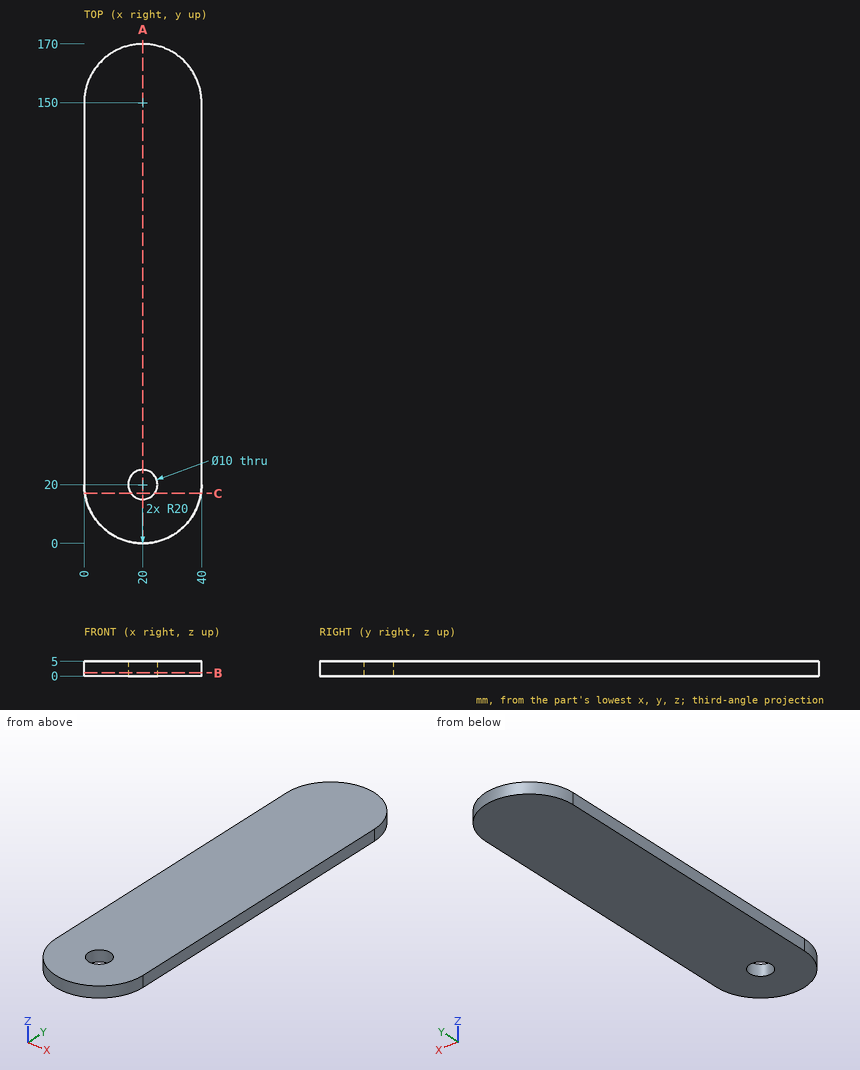
Print and shaded views of the part. All mm, measured from the part's lowest x, y and z. Coordinates: 2 decimals unless noted, no trailing zeros. Loops run counter-clockwise (first coordinate to the right, second up) from the corner with the lowest first, then second, coordinate; pieces in that order, holes last. Notation, with made-up numbers: M 47.5,53.5 L 78.5,53.5 A22 cw 78.5,64.5 Z; hole C 39,1 d1. An arc over 180 degrees is marked long. Use a Markdown table: item, result. Add a question column.
Q1. Cut at C-C (y = 17). Write the cut outline in (x, z), and give its area (3 significant figures).
Q2. Cut at A-A (x = 20). Write the cut outline in (y, z).
Q3. Cut at B-B (z = 1.05). Write the cut outline in (x, y), and give its area (3 significant figures).
Q4. Probe L1, parallel to Y at x = 20, z = 3.3; L2, parallel to Y at x = 18.5, z = 3.55; L3, parallel to Y at x = 38, z = 3.25. List the from-to ranges inside material, lowest first.
Q5. Pin check, flat tips, straight feed: P1, Ø10, axis at x = 29, y = 85, coming from the -Z side; P2, Ø2, axis at x = 19, z = 2.5, coming from the +Y side. Stop position of each tip, or through.
Worked out:
| question | item | result |
|---|---|---|
| 1 | outline | M 0.23,0 L 16,0 L 16,5 L 0.23,5 Z; M 24,0 L 39.77,0 L 39.77,5 L 24,5 Z |
| 1 | area | 158 mm2 |
| 2 | outline | M 0,0 L 15,0 L 15,5 L 0,5 Z; M 25,0 L 170,0 L 170,5 L 25,5 Z |
| 3 | outline | M 0,20 A20 ccw 40,20 L 40,150 A20 ccw 0,150 Z; hole C 20,20 d10 |
| 3 | area | 6,380 mm2 |
| 4 | L1 | y = 0 to 15, 25 to 170 |
| 4 | L2 | y = 0.06 to 15.23, 24.77 to 169.94 |
| 4 | L3 | y = 11.28 to 158.72 |
| 5 | P1 | stops at z = 0 |
| 5 | P2 | stops at y = 170 |
